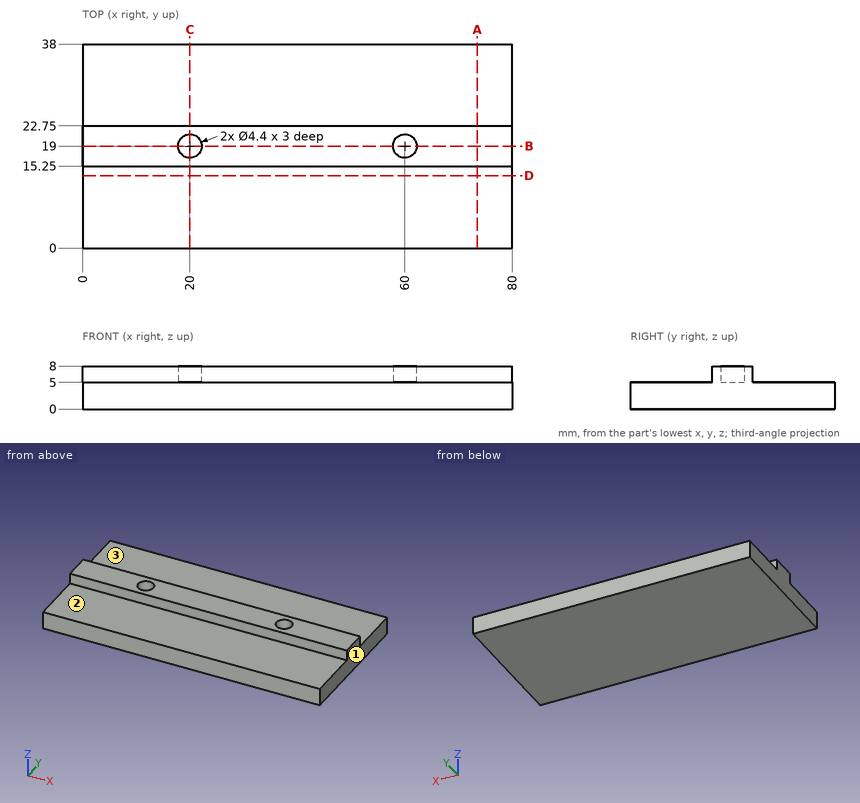
Job drawing, mm, ordinate dimensions from the low corner. One solid piece. A direction names the side the tool comes from. Round coordinates to 2 decimals unless told otherwise and drop trailing zeros. Loops run counter-clockwise (first coordinate to the right, second up) from the corner with the lowest first, then second, coordinate; pieces in that order, holes last.
Item 1: Cut at D-D, the plane y = 13.5. Give the cut face in (x, z), then the cut area to 3 significant figures.
Item 2: 3-axis set-ups, long thin cutter, end or side, ignore diameter. For the marked faces 1, 2 and 3: which of +Z, -Z, +X, -X, +Y, -Y reach the whole face in a straight line?
Item 3: Drop flat-ended pins along their axis: P1, Ø12, axis at x = 23, y = 34, coming from the +Z side; P2, Ø2.5, axis at x = 33, z = 7, coming from the -Y side. Give the stop position or say it passes through.
Item 4: Cut at A-A, the plane x = 73.5. Give the cut face in (y, z).
Item 5: Cut at C-C, the plane x = 20. Give the cut face in (y, z).
Item 6: Cut at B-B, the plane y = 19. Give the cut face in (x, z), then the cut area to 3 significant figures.
Item 7: Drill centre lines: line 1 (X direction, y = 19, z = 6.6); line 2 (Y direction, x = 20, z = 7.3); line 3 (Y direction, x = 10.5, z = 6.25). Where is each one in solid material? Low to high.
A:
1. outline: (0, 0) - (80, 0) - (80, 5) - (0, 5) - close
1. area: 400 mm2
2. face 1: +Z, -Z, +X, +Y, -Y
2. face 2: +Z, +X, -X, -Y
2. face 3: +Z, +X, -X, +Y
3. P1: stops at z = 5
3. P2: stops at y = 15.25
4. outline: (0, 0) - (38, 0) - (38, 5) - (22.75, 5) - (22.75, 8) - (15.25, 8) - (15.25, 5) - (0, 5) - close
5. outline: (0, 0) - (38, 0) - (38, 5) - (22.75, 5) - (22.75, 8) - (21.2, 8) - (21.2, 5) - (16.8, 5) - (16.8, 8) - (15.25, 8) - (15.25, 5) - (0, 5) - close
6. outline: (0, 0) - (80, 0) - (80, 8) - (62.2, 8) - (62.2, 5) - (57.8, 5) - (57.8, 8) - (22.2, 8) - (22.2, 5) - (17.8, 5) - (17.8, 8) - (0, 8) - close
6. area: 614 mm2
7. line 1: x = 0 to 17.8, 22.2 to 57.8, 62.2 to 80
7. line 2: y = 15.25 to 16.8, 21.2 to 22.75
7. line 3: y = 15.25 to 22.75
